Geometry check sheet. Reference: the model listing, model coordinates, mm. Give positions to 0.01 mm unless a question says otherwise; leave off trailing zeros. Write each loop counter-clockwise with the first axis right and the second up, starting at its lowest first coordinate (ties: lowest second). Pieces come first, ordered by that corner, then holes. Notation, with made-up numbers: (10.25, 61) -> (49.25, 61) arc R28 ccw to (49.25, 79) -> close; hole circle Ø3 at (-3, 31.25). An arc over 180 degrees is marked (long way). One line per item, written item: value.
Autodesk Inventor part; units mm, degrees
ref_plane "YZ Plane" through (0, 0, 0) normal (1, 0, 0) x (0, 1, 0)
ref_plane "XZ Plane" through (0, 0, 0) normal (0, 1, 0) x (-1, 0, 0)
ref_plane "XY Plane" through (0, 0, 0) normal (0, 0, 1) x (1, 0, 0)
sketch "Sketch1" plane through (0, 0, 0) normal (0, 1, 0) x (-1, 0, 0)
  circle A0 centre (0, 0) radius 2
  line L0 (3.5, -2.0207) -> (0, -4.0415)
  line L1 (0, -4.0415) -> (-3.5, -2.0207)
  line L2 (-3.5, -2.0207) -> (-3.5, 2.0207)
  line L3 (-3.5, 2.0207) -> (0, 4.0415)
  line L4 (0, 4.0415) -> (3.5, 2.0207)
  line L5 (3.5, 2.0207) -> (3.5, -2.0207)
  dimension "d0" = 4
  dimension "d1" = 3.5
extrude "Extrusion1" add sketch "Sketch1" along normal blind 3
thread "Thread1"
fillet "Fillet1" radius 1 6 edges at (-3.5, 1.5, 2.0207) (0, 1.5, 4.0415) (3.5, 1.5, 2.0207) (3.5, 1.5, -2.0207) (0, 1.5, -4.0415) (-3.5, 1.5, -2.0207)
properties part number "Moer"
1) Sectioned sample at B-B on z = 0. Record the cut outline in (x, y), plus the area to 3 significant figures.
Verdict:
outline: (-3.5, 0) -> (-2, 0) -> (-2, 3) -> (-3.5, 3) -> close; (2, 0) -> (3.5, 0) -> (3.5, 3) -> (2, 3) -> close
area: 9.00 mm^2
2) Mould release check, pull along X, two halves, no side actions. Record for faces 1 (the flat face through (2, 3, -2)), 2 (the flat face through (1.8, 1.5, 3)), 3 (the cylindrical face through (0, 1, 2)), 4 (the cylindrical face through (-3.36, 1.52, -1.95)): released by +X, released by -X, zero draft, split by the parting line, or undercut.
Verdict:
face 1: zero draft
face 2: released by +X
face 3: undercut
face 4: released by -X
3) Sectioned sample at A-A on x = 0. Record the cut outline in (y, z), plus the area to 3 significant figures.
Verdict:
outline: (0, -3.89) -> (3, -3.89) -> (3, -2) -> (0, -2) -> close; (0, 2) -> (3, 2) -> (3, 3.89) -> (0, 3.89) -> close
area: 11.3 mm^2
4) Sectioned sample at C-C on y = 1.45. Record the cut outline in (x, z).
Verdict:
outline: (-3.5, -1.44) arc R1 ccw to (-3, -2.31) -> (-0.5, -3.75) arc R1 ccw to (0.5, -3.75) -> (3, -2.31) arc R1 ccw to (3.5, -1.44) -> (3.5, 1.44) arc R1 ccw to (3, 2.31) -> (0.5, 3.75) arc R1 ccw to (-0.5, 3.75) -> (-3, 2.31) arc R1 ccw to (-3.5, 1.44) -> close; hole circle Ø4 at (0, 0)
5) Sectioned sample at D-D on z = 3.25. Record the cut outline in (x, y).
Verdict:
outline: (-1.37, 0) -> (1.37, 0) -> (1.37, 3) -> (-1.37, 3) -> close
6) Scan lines: probe 1 along Z at (x, y) = (0, 0.7); probe 2 along Z at (x, y) = (-1.25, 0.5); probe 3 along X at (y, z) = (1.85, -1). Record each from-to range of solid material in increasing order.
Verdict:
probe 1: -3.89 to -2, 2 to 3.89
probe 2: -3.32 to -1.56, 1.56 to 3.32
probe 3: -3.5 to -1.73, 1.73 to 3.5
